```python
from build123d import *

# Parameters (mm, degrees)
SKETCH2_R           = 50
SKETCH2_R_2         = 39
BOSS_EXTRUDE1_DEPTH = 5
SKETCH3_R           = 47
SKETCH3_R_2         = 3
SKETCH3_R_3         = 39
BOSS_EXTRUDE2_DEPTH = 4
SKETCH4_R           = 39
SKETCH4_R_2         = 38
BOSS_EXTRUDE3_DEPTH = 1
SKETCH6_R           = 5
SKETCH6_R_2         = 2
BOSS_EXTRUDE4_DEPTH = 5
FILLET1_R           = 5
SKETCH7_R           = 3.6
CUT_EXTRUDE1_DEPTH  = 3
SKETCH8_R           = 3.15
CUT_EXTRUDE2_DEPTH  = 4


with BuildPart() as part:
    # Sketch2 → Boss-Extrude1 (new body)
    with BuildSketch(Plane.XY):
        Circle(SKETCH2_R)
        Circle(SKETCH2_R_2, mode=Mode.SUBTRACT)
    extrude(amount=BOSS_EXTRUDE1_DEPTH)

    # Sketch3 → Boss-Extrude2 (add)
    with BuildSketch(Plane(origin=(0, 0, 0), x_dir=(-1, 0, 0), z_dir=(0, 0, -1))):
        Circle(SKETCH3_R)
        with Locations((-43, 0)):
            Circle(SKETCH3_R_2, mode=Mode.SUBTRACT)
        Circle(SKETCH3_R_3, mode=Mode.SUBTRACT)
        with Locations((-32.939911054, 27.639867217)):
            Circle(SKETCH3_R_2, mode=Mode.SUBTRACT)
        with Locations((-7.46687164, 42.34673338)):
            Circle(SKETCH3_R_2, mode=Mode.SUBTRACT)
        with Locations((21.5, 37.239092363)):
            Circle(SKETCH3_R_2, mode=Mode.SUBTRACT)
        with Locations((40.406782694, 14.706866163)):
            Circle(SKETCH3_R_2, mode=Mode.SUBTRACT)
        with Locations((40.406782694, -14.706866163)):
            Circle(SKETCH3_R_2, mode=Mode.SUBTRACT)
        with Locations((21.5, -37.239092363)):
            Circle(SKETCH3_R_2, mode=Mode.SUBTRACT)
        with Locations((-7.46687164, -42.34673338)):
            Circle(SKETCH3_R_2, mode=Mode.SUBTRACT)
        with Locations((-32.939911054, -27.639867217)):
            Circle(SKETCH3_R_2, mode=Mode.SUBTRACT)
    extrude(amount=BOSS_EXTRUDE2_DEPTH)

    # Sketch4 → Boss-Extrude3 (add)
    with BuildSketch(Plane(origin=(0, 0, -4), x_dir=(-1, 0, 0), z_dir=(0, 0, -1))):
        Circle(SKETCH4_R)
        Circle(SKETCH4_R_2, mode=Mode.SUBTRACT)
    extrude(amount=-BOSS_EXTRUDE3_DEPTH)

    # Sketch6 → Boss-Extrude4 (add)
    with BuildSketch(Plane.XY.offset(5)):
        with Locations((52, 0)):
            Circle(SKETCH6_R)
        with Locations((52, 0)):
            Circle(SKETCH6_R_2, mode=Mode.SUBTRACT)
        with Locations((-52, 0)):
            Circle(SKETCH6_R)
        with Locations((-52, 0)):
            Circle(SKETCH6_R_2, mode=Mode.SUBTRACT)
        with Locations((0, 52)):
            Circle(SKETCH6_R)
        with Locations((0, 52)):
            Circle(SKETCH6_R_2, mode=Mode.SUBTRACT)
        with Locations((0, -52)):
            Circle(SKETCH6_R)
        with Locations((0, -52)):
            Circle(SKETCH6_R_2, mode=Mode.SUBTRACT)
    extrude(amount=-BOSS_EXTRUDE4_DEPTH)

    # Fillet1
    fillet1_edges = [part.edges().sort_by_distance(p)[0] for p in [
        (49.798076923, -4.489046086, 2.5),
        (49.798076923, 4.489046086, 2.5),
        (-49.798076923, 4.489046086, 2.5),
        (-49.798076923, -4.489046086, 2.5),
        (4.489046086, 49.798076923, 2.5),
        (-4.489046086, 49.798076923, 2.5),
        (-4.489046086, -49.798076923, 2.5),
        (4.489046086, -49.798076923, 2.5),
    ]]
    fillet(fillet1_edges, radius=FILLET1_R)

    # Sketch7 → Cut-Extrude1 (cut)
    with BuildSketch(Plane.XY.offset(5)):
        with Locations((52, 0)):
            Circle(SKETCH7_R)
        with Locations((0, 52)):
            Circle(SKETCH7_R)
        with Locations((-52, 0)):
            Circle(SKETCH7_R)
        with Locations((0, -52)):
            Circle(SKETCH7_R)
    extrude(amount=-CUT_EXTRUDE1_DEPTH, mode=Mode.SUBTRACT)

    # Sketch8 → Cut-Extrude2 (cut)
    with BuildSketch(Plane(origin=(0, 0, -4), x_dir=(-1, 0, 0), z_dir=(0, 0, -1))):
        with Locations((-32.939911054, 27.639867217)):
            Circle(SKETCH8_R)
        with Locations((-43, 0)):
            Circle(SKETCH8_R)
        with Locations((-7.46687164, 42.34673338)):
            Circle(SKETCH8_R)
        with Locations((21.5, 37.239092363)):
            Circle(SKETCH8_R)
        with Locations((40.406782694, 14.706866163)):
            Circle(SKETCH8_R)
        with Locations((40.406782694, -14.706866163)):
            Circle(SKETCH8_R)
        with Locations((21.5, -37.239092363)):
            Circle(SKETCH8_R)
        with Locations((-7.46687164, -42.34673338)):
            Circle(SKETCH8_R)
        with Locations((-32.939911054, -27.639867217)):
            Circle(SKETCH8_R)
    extrude(amount=-CUT_EXTRUDE2_DEPTH, mode=Mode.SUBTRACT)


solid = part.part
```
The listing builds one solid part. Answer for the finished solid, in the listing's coordinates (mm). A direction names the side the tool comes from. Give positions to 0.01 mm unless a question says otherwise; leave off trailing zeros. Order: outer loops, then holes, each group sorted by start corner. A loop starts at its lowest first (then second) coordinate and runs counter-clockwise, first axis right, second up.
Item 1: Which of the six approach directions +Z, -Z, +X, -X, +Y, -Y give full straight-line access (tool end or side, diameter ignored) to faces 4 (the face through (-44.83, 14.12, -1.97)), 5 (the face through (35.054, -35.654, 2.465)), 6 (the face through (2, 50, 2))?
From the geometry:
face 4: -Z
face 5: +Z, -Z, +X, -Y
face 6: +Z
Item 2: For a pull along X with two mould halves and no side action, classify faces 1 (the face through (0, 57, 3)), 2 (the face through (4, -38, -4)), 3 (the face through (-37.9, 12.8, -2)) as pulls with the +X half, pulls with the -X half, needs draft (parallel to the pull), parting line crosses it, or undercut.
From the geometry:
face 1: parting line crosses it
face 2: needs draft
face 3: undercut
Item 3: Given pin 1 Ø1.8 at (x, y) = (-40.5, 14) entering from -Z; pin 2 Ø6 at (x, y) = (52, 0) entering from +Z; pin 3 Ø3 at (y, z) = (5.5, 1.5) entering from +X, each flat-ended and moving along its own axis, determine where each tip first touches the part or whether it passes through.
From the geometry:
pin 1: stops at z = 0
pin 2: stops at z = 2
pin 3: stops at x = 55
Item 4: The part is cut by section A-A, the plane y = -22. Give the vertices of the cut face in (x, z).
From the geometry:
outline: (-44.9, 0) - (-41.53, 0) - (-41.53, -4) - (-30.98, -4) - (-30.98, -3) - (-32.2, -3) - (-32.2, 5) - (-44.9, 5) - close; (30.98, -4) - (41.53, -4) - (41.53, 0) - (44.9, 0) - (44.9, 5) - (32.2, 5) - (32.2, -3) - (30.98, -3) - close
Item 5: The part is cut by section B-B, the plane y = 0. Count the separate pieces of the cut face and the enclosed holes in it, and give its area (3 significant figures).
From the geometry:
separate pieces: 4
enclosed holes: 0
area: 162 mm2
Item 6: Find the intervals of material crossed by probe 1 along Y at (x, z) = (0, 1.45); probe 2 along Y at (x, z) = (0, 4.15); probe 3 along Y at (x, z) = (0, -1.25), in increasing order.
From the geometry:
probe 1: y = -57 to -54, -50 to -39, 39 to 50, 54 to 57
probe 2: y = -57 to -55.6, -48.4 to -39, 39 to 48.4, 55.6 to 57
probe 3: y = -47 to -39, 39 to 47
